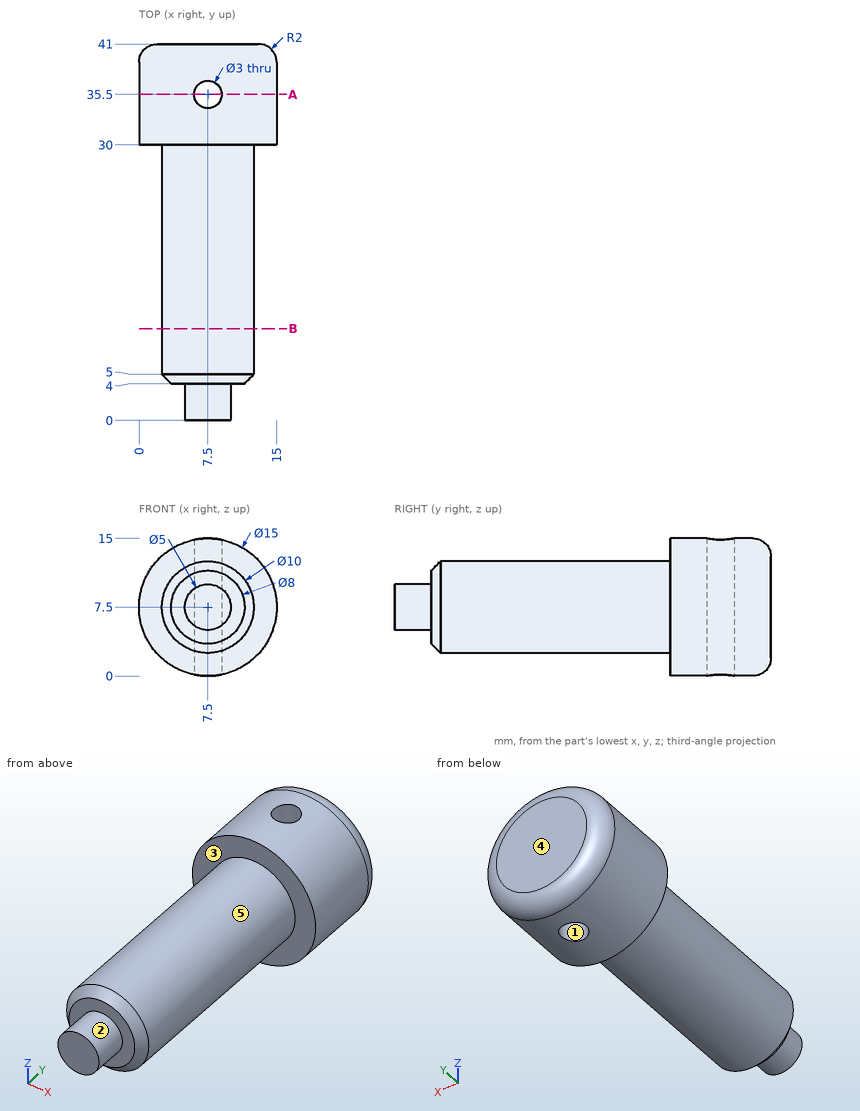
Check sheet for the drawn part. Datum: minimum x, y, z corner. Units: mm. A direction names the side the tool comes from. Round coordinates to 2 decimals unless told otherwise and drop trailing zeros. Write each loop counter-clockwise with the first axis right and the second up, starting at its lowest first coordinate (ties: lowest second). Pieces come first, ordered by that corner, then holes. Notation, with made-up numbers: (32.25, -12) -> (79.25, -12) arc R11 ccw to (79.25, 3) -> close; hole circle Ø8 at (15.5, -33). An arc over 180 degrees is marked (long way). One line per item, written item: value. Start each with the question number.
(1) Cross-section at B-B, the plane y = 10. Record the cut outline in (x, z).
(2) Access from +Z, -Z, +X, -X, +Y, -Y to the whole of each face (thin tool, end or side, straight path). Record for the marked faces 4 and 5.
(3) Scan lines: line 1 (Y direction, x = 7.5, z = 8); line 2 (X direction, y = 36.5, z = 3.25); line 3 (Y direction, x = 4.75, z = 6.75). Record each from-to range of solid material in increasing order. Write a range as [from, to].
(4) Cross-section at A-A, the plane y = 35.5. Record the cut outline in (x, z).
(5) Go/stop test with flat-tipped pins: pin 1 Ø2 at (x, y) = (5, 23) entering from +Z; pin 2 Ø5 at (y, z) = (22.5, 4) entering from +X; pin 3 Ø4 at (y, z) = (12, 10) entering from +X. Record where each tip stops, or that it passes through.
(6) Draft check along X on the marked faces 1, 2 and 3. Enter one of: +X half, -X half, draft (parallel to the pull), parting line (faces both ways), or undercut.
Answer:
1. outline: circle Ø10 at (7.5, 7.5)
2. face 4: +Z, -Z, +X, -X, +Y
2. face 5: -Y
3. line 1: [0, 34], [37, 41]
3. line 2: [1.32, 6.38], [8.62, 13.68]
3. line 3: [4, 41]
4. outline: (6, 0.15) -> (6, 14.85) arc R7.5 ccw to start; (9, 0.15) arc R7.5 ccw to (9, 14.85) -> close
5. pin 1: z = 12.27
5. pin 2: x = 12.4
5. pin 3: x = 12.47
6. face 1: undercut
6. face 2: parting line
6. face 3: draft
